from build123d import *

# Parameters (mm, degrees)
SKETCH1_R          = 100
BODY_DEPTH         = 83.89
SKETCH2_R          = 20.985
SHAFT_DEPTH        = 80.18
MOUNT_START        = -6.309503
SKETCH5_W          = 30
SKETCH5_H          = 20
MOUNT_BASE_DEPTH   = 51.309503
SKETCH6_W          = 30
SKETCH6_H          = 20
SKETCH6_W_2        = 24
SKETCH6_H_2        = 14
MOUNT_TONGUE_DEPTH = 35
MOUNT_HOLES_REACH  = 208.935
SKETCH7_R          = 5


with BuildPart() as part:
    # Sketch1 → Body (new body)
    with BuildSketch(Plane.XY):
        Circle(SKETCH1_R)
    extrude(amount=BODY_DEPTH)

    # Sketch2 → Shaft (add)
    with BuildSketch(Plane.XY):
        Circle(SKETCH2_R)
    extrude(amount=-SHAFT_DEPTH)

    # Sketch5 → Mount Base (add)
    with BuildSketch(Plane(origin=(0, 20.985, 0), x_dir=(1, 0, 0), z_dir=(0, 1, 0)).offset(MOUNT_START)):
        with Locations((0, 60.18)):
            Rectangle(SKETCH5_W, SKETCH5_H)
    extrude(amount=MOUNT_BASE_DEPTH)

    # Sketch6 → Mount Tongue (cut)
    with BuildSketch(Plane(origin=(0, 65.985, 0), x_dir=(1, 0, 0), z_dir=(0, 1, 0))):
        with Locations((0, 60.18)):
            Rectangle(SKETCH6_W, SKETCH6_H)
        with Locations((0, 60.18)):
            Rectangle(SKETCH6_W_2, SKETCH6_H_2, mode=Mode.SUBTRACT)
    extrude(amount=-MOUNT_TONGUE_DEPTH, mode=Mode.SUBTRACT)

    # Sketch7 → Mount Holes (cut, up to next)
    with BuildSketch(Plane(origin=(0, 0, -67.18), x_dir=(-1, 0, 0), z_dir=(0, 0, -1)), mode=Mode.PRIVATE) as mount_holes_sk1:
        with Locations((0, 40.985)):
            Circle(SKETCH7_R)
    mount_holes_tool1 = extrude(mount_holes_sk1.sketch, amount=-MOUNT_HOLES_REACH, mode=Mode.PRIVATE) & part.part
    # Sketch7 → Mount Holes (cut, up to next)
    with BuildSketch(Plane(origin=(0, 0, -67.18), x_dir=(-1, 0, 0), z_dir=(0, 0, -1)), mode=Mode.PRIVATE) as mount_holes_sk2:
        with Locations((0, 55.985)):
            Circle(SKETCH7_R)
    mount_holes_tool2 = extrude(mount_holes_sk2.sketch, amount=-MOUNT_HOLES_REACH, mode=Mode.PRIVATE) & part.part
    add(mount_holes_tool1.solids().sort_by_distance((0, 40.985, -67.18))[0], mode=Mode.SUBTRACT)
    add(mount_holes_tool2.solids().sort_by_distance((0, 55.985, -67.18))[0], mode=Mode.SUBTRACT)


solid = part.part
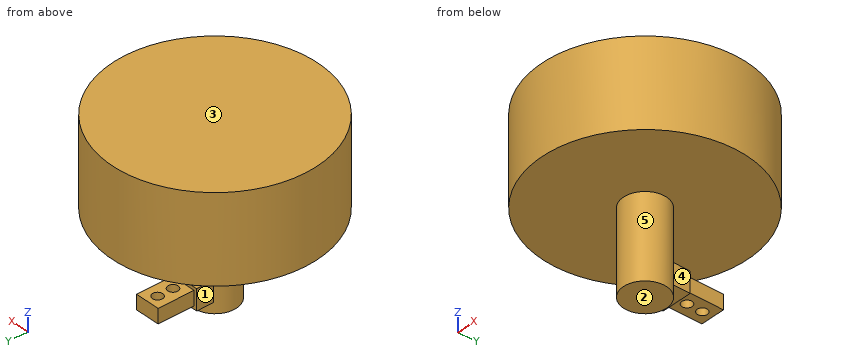
Build history of the part. All positions in model axes, mm. Face numbers are marked on the shaded views. A direction names the side the tool comes from. Round coordinates to 2 decimals unless told otherwise and drop trailing zeros. Write each loop counter-clockwise with the first axis right and the second up, starting at its lowest first coordinate (ties: lowest second). Pieces come first, ordered by that corner, then holes. Notation, with made-up numbers: M -29.75,-8 L -21.75,-8 A29 cw -21.75,14 Z; hole C -13.75,-6 d5. An arc over 180 degrees is marked long. Answer as a JSON object with one key per item and string values. Group by question number.
(1) Cut at B-B (z = -64). Give the cut face in (x, y) (1 decimal), and give its area (3 significant figures).
(2) Cut at D-D (z = 20.5). Give the cut face in (x, y), and give its area (3 significant figures).
(3) Mould opens along Z. For the marked faces 3, 4 and 5 say: pulls with the +Z half, pulls with the -Z half, needs draft (parallel to the pull), parting line crosses it, or undercut.
(4) Which spindle directions (+Z, -Z, +X, -X, +Y, -Y) get a long thin tool onto all of the face, cutting with end or side? Do the marked faces 1 and 2. Say none if no direction does.
(5) Flat gauge pins, fed straight in: pin 1 (1.5 mm diameter, centred on x = 7, y = 56, fed in from -Z); pin 2 (5 mm diameter, centred on x = 22.5, z = 6.5, fed in from -Y); pin 3 (22 mm diameter, centred on x = 1.5, z = -61, fed in from +Y) (3 decimals). Where does each tip first touch, or does it go through?
(6) Cut at A-A (x = 0). Give the cut face in (y, z) (3 decimals).
(7) Cut at C-C (y = 0). Give the cut face in (x, z) (3 decimals).
(8) Drill centre lines: L1, parallel to Y at x = 0, z = -63.5 (3 decimals); L2, parallel to Z at x = -22, y = 84; L3, parallel to Z at x = 10, y = 25.5. Where is each one in solid material? Low to high.
Responses:
{
 "1": {"outline": "M -15,14.7 A21 ccw long 15,14.7 L 15,31 L 12,31 L 12,66 L -12,66 L -12,31 L -15,31 Z; hole C 0,41 d10; hole C 0,56 d10", "area": "2,430 mm2"},
 "2": {"outline": "C 0,0 d200", "area": "31,400 mm2"},
 "3": {"face 3": "pulls with the +Z half", "face 4": "needs draft", "face 5": "undercut"},
 "4": {"face 1": "-Z, -X, +Y", "face 2": "-Z, +X, -X, +Y, -Y"},
 "5": {"pin 1": "stops at z = -67.18", "pin 2": "stops at y = -97.98", "pin 3": "stops at y = 65.985"},
 "6": {"outline": "M -100,0 L -20.985,0 L -20.985,-80.18 L 20.985,-80.18 L 20.985,-70.18 L 30.985,-70.18 L 30.985,-67.18 L 35.985,-67.18 L 35.985,-53.18 L 30.985,-53.18 L 30.985,-50.18 L 20.985,-50.18 L 20.985,0 L 100,0 L 100,83.89 L -100,83.89 Z; M 45.985,-67.18 L 50.985,-67.18 L 50.985,-53.18 L 45.985,-53.18 Z; M 60.985,-67.18 L 65.985,-67.18 L 65.985,-53.18 L 60.985,-53.18 Z"},
 "7": {"outline": "M -100,0 L -20.985,0 L -20.985,-80.18 L 20.985,-80.18 L 20.985,0 L 100,0 L 100,83.89 L -100,83.89 Z"},
 "8": {"L1": "y = -20.985 to 35.985, 45.985 to 50.985, 60.985 to 65.985", "L2": "z = 0 to 83.89", "L3": "z = -70.18 to -50.18, 0 to 83.89"}
}
